Geometry: final body of the model. Coordinates: model frame, mm. A direction names the side the tool comes from. Round coordinates to 2 decimals unless told otherwise and drop trailing zeros. Write each loop counter-clockwise with the first axis right and the second up, starting at its lowest first coordinate (ties: lowest second). Pieces come first, ordered by that corner, then holes.
from build123d import *

# Parameters (mm, degrees)
F1_DEPTH = 5
F2_R     = 1
F3_DEPTH = 25
F4_R     = 1
F5_DEPTH = 25
F6_R     = 4.99999
F7_R     = 5


# Not quite as in the source:
# - a fillet or chamfer is up to 0.001 mm smaller than in the source, because OpenCascade refuses the exact size
# - a feature names something its author has since deleted; it is built from what else it names


with BuildPart() as f1:
    # F0 (on Front) → F1 (new body, symmetric)
    with BuildSketch(Plane.XZ):
        with BuildLine():
            ThreePointArc((4.105083276, -3.0262668912), (2.2995694004, -4.5521402189), (0, -5.1))
            Line((0, -5.1), (0, -8))
            ThreePointArc((0, -8), (3.9939571451, -6.9316885622), (6.9212167652, -4.0120765807))
            Line((6.9212167652, -4.0120765807), (4.105083276, -3.0262668912))
        make_face()
        with BuildLine():
            ThreePointArc((5.0962805256, -0.1947429178), (4.8135907549, -1.6850353244), (4.105083276, -3.0262668912))
            Line((4.105083276, -3.0262668912), (6.9212167652, -4.0120765807))
            ThreePointArc((6.9212167652, -4.0120765807), (7.5507305959, -2.6431926657), (7.9124140148, -1.1805526072))
            Line((7.9124140148, -1.1805526072), (5.0962805256, -0.1947429178))
        make_face()
        with BuildLine():
            ThreePointArc((2, 4.6914816423), (4.3079109714, 2.7298174046), (5.0962805256, -0.1947429178))
            Line((5.0962805256, -0.1947429178), (7.9124140148, -1.1805526072))
            ThreePointArc((7.9124140148, -1.1805526072), (7.4476378384, 2.9210769638), (5, 6.2449979984))
            ThreePointArc((5, 6.2449979984), (3.5795567819, 7.1544932207), (2, 7.7459666924))
            Line((2, 7.7459666924), (2, 4.6914816423))
        make_face()
        with BuildLine():
            ThreePointArc((7.9124140148, -1.1805526072), (7.5507305959, -2.6431926657), (6.9212167652, -4.0120765807))
            Line((6.9212167652, -4.0120765807), (19.4194533219, -8.3871826424))
            Line((19.4194533219, -8.3871826424), (20.4106505716, -5.555658669))
            Line((20.4106505716, -5.555658669), (7.9124140148, -1.1805526072))
        make_face()
        with BuildLine():
            Line((2, 15), (2, 7.7459666924))
            ThreePointArc((2, 7.7459666924), (3.5795567819, 7.1544932207), (5, 6.2449979984))
            Line((5, 6.2449979984), (5, 15))
            Line((5, 15), (2, 15))
        make_face()
    extrude(amount=F1_DEPTH, both=True)

    # F2 (on face) → F3 (cut)
    with BuildSketch(Plane(origin=(0.4955986248, 0, 1.4157619867), x_dir=(0.9438413245, 0, -0.3303990832), z_dir=(0.3303990832, 0, 0.9438413245))):
        with Locations((16.1, 0)):
            Circle(F2_R)
    extrude(amount=-F3_DEPTH, mode=Mode.SUBTRACT)

    # F4 (on face) → F5 (cut)
    with BuildSketch(Plane.YZ.offset(5)):
        with Locations((0, 10.6224989992)):
            Circle(F4_R)
    extrude(amount=-F5_DEPTH, mode=Mode.SUBTRACT)

    # F6 (radius 5 in the source; OpenCascade refuses exactly that, so slightly less here)
    f6_edges = [f1.edges().sort_by_distance(p)[0] for p in [
        (19.915052, 5, -6.971421),
        (19.915052, -5, -6.971421),
        (3.5, -5, 15),
        (3.5, 5, 15),
    ]]
    fillet(f6_edges, radius=F6_R)

    # F7
    f7_edges = [f1.edges().sort_by_distance(p)[0] for p in [
        (5, 0, 6.244998),
        (7.912414, 0, -1.180553),
        (6.921217, 0, -4.012077),
    ]]
    fillet(f7_edges, radius=F7_R)

    # F8: F1 across plane


with BuildPart() as f1_1:
    add(f1.part)
    add(f1.part.mirror(Plane.YZ))


solid = f1_1.part
1) First-contact query: P1, Ø2, axis at y = -2.5, z = -1, coming from the -X side; P2, Ø2.5, axis at y = 0, z = 10.62, coming from the +X side; P3, Ø3, axis at y = -1.5, z = 8.5, coming from the +X side. Flat tips, straight axial feed; report the tip coordinate or a pass-through.
2) Reachability of faces 4 (the flat face through (14.71, -1.18, -6.74)), 5 (the flat face through (5, 1, 12)), 6 (the flat face through (2, 0, 9)) from +Z, -Z, +X, -X, +Y, -Y: full face, straight path, thin tool, end or side. Return the list, or none.
3) Section A-A on z = 2.5. Output: boundary loops of the cut face in (x, y).
4) Section D-D on z = 5.5. Output: boundary loops of the cut face in (x, y).
5) Section C-C on y = -1.5. Output: boundary loops of the cut face in (x, z).
6) Draft query along X for faces 1 (the flat face through (-14.8, 1.04, -3.59)), 2 (the cylindrical face through (14.26, 0.04, -4.97)), 3 (the cylindrical face through (-3, -4, 13)). Return one class per face: pulls with the +X half, pulls with the -X half, needs draft (parallel to the pull), parting line crosses it, or undercut.
7) Line query: probe 1 along X at (y, z) = (0.75, 9.5); probe 2 along Z at (x, y) = (3.3, 0); probe 3 along Y at (x, z) = (-15, -5.75). Output: solid intervals per line, ascending.
8) Section B-B on x = -3. State how many separate pieces and enclosed holes the cut face has, plus the area to 3 significant figures.
Filled in:
1. P1: stops at x = -10.43
1. P2: stops at x = 5
1. P3: stops at x = 5.17
2. face 4: -Z, +Y, -Y
2. face 5: +Z, +X, +Y, -Y
2. face 6: +Z, +Y, -Y
3. outline: (-7.6, -5) - (-4.45, -5) - (-4.45, 5) - (-7.6, 5) - close; (4.45, -5) - (7.6, -5) - (7.6, 5) - (4.45, 5) - close
4. outline: (-5.86, -5) - (-2, -5) - (-2, 5) - (-5.86, 5) - close; (2, -5) - (5.86, -5) - (5.86, 5) - (2, 5) - close
5. outline: (-20.19, -5.48) - (-19.2, -8.31) - (-10.13, -5.14) arc R5 cw to (-5.22, -6.06) arc R8 ccw to (5.22, -6.06) arc R5 cw to (10.13, -5.14) - (19.2, -8.31) - (20.19, -5.48) - (11.12, -2.3) arc R5 cw to (7.86, 1.49) arc R8 ccw to (6.15, 5.11) arc R5 cw to (5, 8.31) - (5, 14.77) - (2, 14.77) - (2, 4.69) arc R5.1 cw (long way) to (-2, 4.69) - (-2, 14.77) - (-5, 14.77) - (-5, 8.31) arc R5 cw to (-6.15, 5.11) arc R8 ccw to (-7.86, 1.49) arc R5 cw to (-11.12, -2.3) - close
6. face 1: pulls with the -X half
6. face 2: undercut
6. face 3: needs draft
7. probe 1: x = -5 to -2, 2 to 5
7. probe 2: z = -7.29 to -3.89, 3.89 to 9.62, 11.62 to 15
7. probe 3: y = -5 to -1, 1 to 5
8. separate pieces: 2
8. enclosed holes: 1
8. area: 128 mm2
